```python
from build123d import *

# Parameters (mm, degrees)
F0_W     = 25.4
F0_H     = 50.8
F0_W_2   = 19.05
F0_H_2   = 44.45
F1_DEPTH = 152.4
F2_R     = 3.175
F3_R     = 1.524


with BuildPart() as f1:
    # F0 (on Front) → F1 (new body)
    with BuildSketch(Plane.XZ):
        with Locations((-6.305698, 2.473545)):
            Rectangle(F0_W, F0_H)
        with Locations((-6.305698, 2.473545)):
            Rectangle(F0_W_2, F0_H_2, mode=Mode.SUBTRACT)
    extrude(amount=F1_DEPTH)

    # F2
    f2_edges = [f1.edges().sort_by_distance(p)[0] for p in [
        (-19.005698, -76.2, 27.873545),
        (6.394302, -76.2, 27.873545),
        (-19.005698, -76.2, -22.926455),
        (6.394302, -76.2, -22.926455),
    ]]
    fillet(f2_edges, radius=F2_R)

    # F3
    f3_edges = [f1.edges().sort_by_distance(p)[0] for p in [
        (-15.830698, -76.2, 24.698545),
        (3.219302, -76.2, 24.698545),
        (3.219302, -76.2, -19.751455),
        (-15.830698, -76.2, -19.751455),
    ]]
    fillet(f3_edges, radius=F3_R)


solid = f1.part
```
CAD build for the part. Positions are in the model's coordinates, mm. A direction names the side the tool comes from. Give positions to 0.01 mm unless a question says otherwise; leave off trailing zeros. Loops run counter-clockwise (first coordinate to the right, second up) from the corner with the lowest first, then second, coordinate; pieces in that order, holes last. Notation, with made-up numbers: (-10, 79.5) -> (42, 79.5) arc R30 cw to (42, 116.5) -> close; hole circle Ø7 at (-5, -13). An arc over 180 degrees is marked (long way). Use a Markdown table: item, result.
1. Which spindle directions (+Z, -Z, +X, -X, +Y, -Y) get a long thin tool onto all of the face, cutting with end or side? Do faces 1 (the flat face through (-15.831, -75, 2)), 2 (the flat face through (4, 0, 3)). Say none if no direction does.
Check result:
| item | result |
|---|---|
| face 1 | +Y, -Y |
| face 2 | +Z, -Z, +X, -X, +Y |
2. Slice it at A-A (z = -0.5). List the corners of the cut face in (x, y), plus the area to 3 significant figures.
Check result:
| item | result |
|---|---|
| outline | (-19.01, -152.4) -> (-15.83, -152.4) -> (-15.83, 0) -> (-19.01, 0) -> close; (3.22, -152.4) -> (6.39, -152.4) -> (6.39, 0) -> (3.22, 0) -> close |
| area | 968 mm^2 |
3. Wall check: L1, parallel to X at y = -9, z = 19.5; L2, parallel to Z at x = -8.25, y = -87; L3, parallel to Z at x = -14.5, y = -39.5. Give the ranges that are in metal, low to high. Write a range as [from, to].
Check result:
| item | result |
|---|---|
| L1 | x = [-19.01, -15.83], [3.22, 6.39] |
| L2 | z = [-22.93, -19.75], [24.7, 27.87] |
| L3 | z = [-22.93, -19.74], [24.69, 27.87] |
4. Slice it at B-B (x = -9.25). List the corners of the cut face in (y, z).
Check result:
| item | result |
|---|---|
| outline | (-152.4, -22.93) -> (0, -22.93) -> (0, -19.75) -> (-152.4, -19.75) -> close; (-152.4, 24.7) -> (0, 24.7) -> (0, 27.87) -> (-152.4, 27.87) -> close |
5. Slice it at C-C (y = -122). List the corners of the cut face in (x, z) (3 decimals), plus the area to 3 significant figures.
Check result:
| item | result |
|---|---|
| outline | (-19.006, -19.751) arc R3.175 ccw to (-15.831, -22.926) -> (3.219, -22.926) arc R3.175 ccw to (6.394, -19.751) -> (6.394, 24.699) arc R3.175 ccw to (3.219, 27.874) -> (-15.831, 27.874) arc R3.175 ccw to (-19.006, 24.699) -> close; hole (-15.831, -18.227) arc R1.524 ccw to (-14.307, -19.751) -> (1.695, -19.751) arc R1.524 ccw to (3.219, -18.227) -> (3.219, 23.175) arc R1.524 ccw to (1.695, 24.699) -> (-14.307, 24.699) arc R1.524 ccw to (-15.831, 23.175) -> close |
| area | 437 mm^2 |
6. Mould opens along X. For faces 3 (the cylindrical face through (5.44, -77.27, -22.02)), 4 (the flat face through (-6, -75, -19.751)), 5 (the flat face through (-19.006, -75, 2)) say: pulls with the +X half, pulls with the -X half, needs draft (parallel to the pull), parting line crosses it, or undercut.
Check result:
| item | result |
|---|---|
| face 3 | pulls with the +X half |
| face 4 | undercut |
| face 5 | pulls with the -X half |
